Check sheet for the modelled part. Datum: model origin and axes. Units: mm. Face numbers are marked on the shaded views. A direction names the side the tool comes from. Round coordinates to 2 decimals unless told otherwise and drop trailing zeros. Loops run counter-clockwise (first coordinate to the right, second up) from the corner with the lowest first, then second, coordinate; pieces in that order, holes last. Notation, with made-up numbers: (62, -12.75) -> (81, -12.75) arc R9 cw to (81, -1.75) -> close; hole circle Ø7 at (-7, 46). An arc over 180 degrees is marked (long way). Use one line per item in the form item = value. Start each with the question number.
(1) Set-up check for the marked faces 5, 6 and 7: record each of +Z, -Z, +X, -X, +Y, -Y from which the full face is reachable in a straight line by a thin tool's end or side.
(2) Sectioned sample at B-B (x = 32.5). Record the cut outline in (y, z), and give its area (3 significant figures).
(3) Sectioned sample at D-D (x = 164). Record the cut outline in (y, z).
(4) Draft check along Y on the marked faces 1, 2, 3 and 4. Enter one of: released by +Y, released by -Y, zero draft, split by the parting line, or undercut.
(5) Sectioned sample at A-A (y = -140). Record the cut outline in (x, z), and give its area (3 significant figures).
(6) Material ranges on probe 1 along Y at (x, z) = (14.5, 33); probe 2 along Y at (x, z) = (32, 3); probe 3 along Y at (x, z) = (32, 5), recorded low to high. Write a range as [from, to].
(7) Go/stop test with flat-tipped pins: pin 1 (1 mm diameter, centred on x = 98.5, y = 131, fed in from -Z); pin 2 (8 mm diameter, centred on x = 173.5, z = 56, fed in from -Y); pin 3 (2 mm diameter, centred on x = 35, z = 63, fed in from +Y); pin 4 (3 mm diameter, centred on x = 47.5, z = 51.5, fed in from +Y). Record where each tip stops, or that it passes through.
(8) Sectioned sample at C-C (z = 116.5). Record the cut outline in (x, y).
from build123d import *

# Parameters (mm, degrees)
BOSS_EXTRUDE1_DEPTH     = 240
SKETCH2_R               = 12.5
CUT_EXTRUDE1_DEPTH      = 133
CUT_EXTRUDE1_DEPTH_BACK = 11
FILLET1_R               = 20


with BuildPart() as part:
    # Sketch1 → Boss-Extrude1 (new body)
    with BuildSketch(Plane.YZ):
        with BuildLine():
            Line((164, 0), (95, 0))
            ThreePointArc((95, 0), (84.393398282, 4.393398282), (80, 15))
            Line((80, 15), (80, 52))
            ThreePointArc((80, 52), (0, 132), (-80, 52))
            Line((-80, 52), (-80, 15))
            ThreePointArc((-80, 15), (-84.393398282, 4.393398282), (-95, 0))
            Line((-95, 0), (-164, 0))
            Line((-164, 0), (-164, 10))
            Line((-164, 10), (-95, 10))
            ThreePointArc((-95, 10), (-91.464466094, 11.464466094), (-90, 15))
            Line((-90, 15), (-90, 52))
            ThreePointArc((-90, 52), (0, 142), (90, 52))
            Line((90, 52), (90, 15))
            ThreePointArc((90, 15), (91.464466094, 11.464466094), (95, 10))
            Line((95, 10), (164, 10))
            Line((164, 10), (164, 0))
        make_face()
    extrude(amount=BOSS_EXTRUDE1_DEPTH)

    # Sketch2 → Cut-Extrude1 (cut, two sides)
    with BuildSketch(Plane.XY.offset(10)) as cut_extrude1_sk:
        with Locations((32.5, 140)):
            Circle(SKETCH2_R)
        with Locations((207.5, 140)):
            Circle(SKETCH2_R)
        with Locations((207.5, -140)):
            Circle(SKETCH2_R)
        with Locations((32.5, -140)):
            Circle(SKETCH2_R)
    extrude(amount=CUT_EXTRUDE1_DEPTH, mode=Mode.SUBTRACT)
    extrude(cut_extrude1_sk.sketch, amount=-CUT_EXTRUDE1_DEPTH_BACK, mode=Mode.SUBTRACT)

    # Fillet1
    fillet1_edges = [part.edges().sort_by_distance(p)[0] for p in [
        (0, -164, 5),
        (0, 164, 5),
        (240, -164, 5),
        (240, 164, 5),
    ]]
    fillet(fillet1_edges, radius=FILLET1_R)


solid = part.part
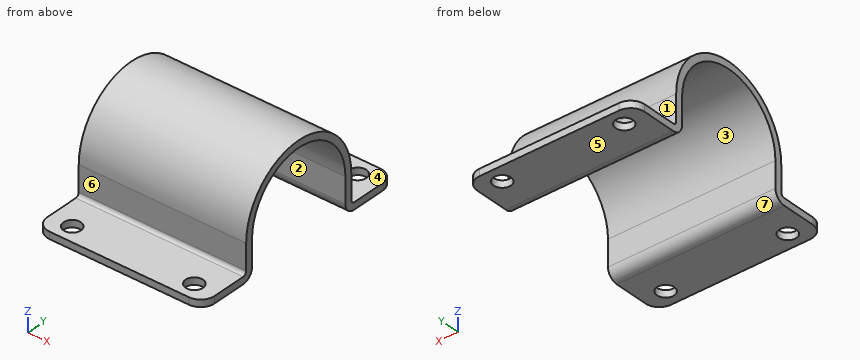
Checks:
q1.face_5 = -Z, +X, -X, +Y, -Y
q1.face_6 = +Z, +X, -X, -Y
q1.face_7 = -Z, +X, -X
q2.outline = (-164, 0) -> (-152.5, 0) -> (-152.5, 10) -> (-164, 10) -> close; (-127.5, 0) -> (-95, 0) arc R15 ccw to (-80, 15) -> (-80, 52) arc R80 cw to (80, 52) -> (80, 15) arc R15 ccw to (95, 0) -> (127.5, 0) -> (127.5, 10) -> (95, 10) arc R5 cw to (90, 15) -> (90, 52) arc R90 ccw to (-90, 52) -> (-90, 15) arc R5 cw to (-95, 10) -> (-127.5, 10) -> close; (152.5, 0) -> (164, 0) -> (164, 10) -> (152.5, 10) -> close
q2.area = 4,600 mm2
q3.outline = (-164, 0) -> (-95, 0) arc R15 ccw to (-80, 15) -> (-80, 52) arc R80 cw to (80, 52) -> (80, 15) arc R15 ccw to (95, 0) -> (164, 0) -> (164, 10) -> (95, 10) arc R5 cw to (90, 15) -> (90, 52) arc R90 ccw to (-90, 52) -> (-90, 15) arc R5 cw to (-95, 10) -> (-164, 10) -> close
q4.face_1 = released by +Y
q4.face_2 = undercut
q4.face_3 = undercut
q4.face_4 = zero draft
q5.outline = (0, 0) -> (20, 0) -> (20, 10) -> (0, 10) -> close; (45, 0) -> (195, 0) -> (195, 10) -> (45, 10) -> close; (220, 0) -> (240, 0) -> (240, 10) -> (220, 10) -> close
q5.area = 1,900 mm2
q6.probe_1 = [-90, -80], [80, 90]
q6.probe_2 = [-164, -152.49], [-127.51, -86], [86, 127.51], [152.49, 164]
q6.probe_3 = [-164, -152.49], [-127.51, -83.82], [83.82, 127.51], [152.49, 164]
q7.pin_1 = 0
q7.pin_2 = -90
q7.pin_3 = 89.44
q7.pin_4 = 90
q8.outline = (0, -62.77) -> (240, -62.77) -> (240, -47.33) -> (0, -47.33) -> close; (0, 47.33) -> (240, 47.33) -> (240, 62.77) -> (0, 62.77) -> close
